Part model, mm, in its own coordinate system. Face numbers are marked on the shaded views. Round coordinates to 2 decimals unless told otherwise and drop trailing zeros. Order: outer loops, then holes, each group sorted by start corner. A loop starts at its lowest first (then second) coordinate and runs counter-clockwise, first axis right, second up. Notation, with made-up numbers: M 74.5,48.25 L 106.5,48.25 A15 ccw 106.5,66.25 Z; hole C 73,-15 d3. An arc over 180 degrees is marked long. Write each question's results on one line, items separated by ' | '. Start each with the question number.
1. Band-saw the part on C-C, the plane x = -30. List the corners of the cut face in (y, z) (3 decimals).
2. Probe L1, parallel to Y at x = 54.25, z = 6; L2, parallel to X at y = 16, z = 8; L3, parallel to Y at x = -25, z = 9. List the from-to ranges inside material, lowest first. Write a range as [from, to].
3. Two-plate mould, pull along Y, no slides. Class the marked faces 1, 2, 3 and 4: +Y half, -Y half, draft (parallel to the pull), parting line (faces both ways), or undercut.
4. Band-saw the part on A-A, the plane x = 55. List the corners of the cut face in (y, z), then the cut area to 3 significant figures.
5. Drop flat-ended pins along their axis: pin 1 Ø3 at (y, z) = (-20, 6.5) entering from +X; pin 2 Ø1 at (y, z) = (18, 10) entering from -X; pin 3 Ø0.9 at (x, z) = (-30, 6.5) entering from +Y. Give the stop position or say it passes through.
6. Band-saw the part on D-D, the plane z = 10.25. List the corners of the cut face in (x, y).
```python
from build123d import *

# Parameters (mm, degrees)
SKETCH1_W           = 130
SKETCH1_H           = 60
SKETCH1_R           = 8
SKETCH1_R_2         = 3.25
BOSS_EXTRUDE1_DEPTH = 12
FILLET1_R           = 6
SKETCH2_R           = 3
SKETCH2_R_2         = 2.5
CUT_EXTRUDE1_DEPTH  = 20
SKETCH3_R           = 3
SKETCH3_R_2         = 1.5
CUT_EXTRUDE2_DEPTH  = 15


with BuildPart() as part:
    # Sketch1 → Boss-Extrude1 (new body)
    with BuildSketch(Plane.XY):
        Rectangle(SKETCH1_W, SKETCH1_H)
        with Locations((-25, 0)):
            Circle(SKETCH1_R, mode=Mode.SUBTRACT)
        with Locations((-5.554563517, 19.445436483)):
            Circle(SKETCH1_R_2, mode=Mode.SUBTRACT)
        with Locations((-44.445436483, 19.445436483)):
            Circle(SKETCH1_R_2, mode=Mode.SUBTRACT)
        with Locations(Location((-44.445436483, -19.445436483, 0), (0, 0, 180))):
            Circle(SKETCH1_R_2, mode=Mode.SUBTRACT)
        with Locations(Location((-5.554563517, -19.445436483, 0), (0, 0, 180))):
            Circle(SKETCH1_R_2, mode=Mode.SUBTRACT)
    extrude(amount=BOSS_EXTRUDE1_DEPTH)

    # Fillet1
    fillet1_edges = [part.edges().sort_by_distance(p)[0] for p in [
        (-65, 0, 0),
        (-65, 0, 12),
    ]]
    fillet(fillet1_edges, radius=FILLET1_R - 0.0001)  # a hair under: the kernel refuses the full size

    # Sketch2 → Cut-Extrude1 (cut)
    with BuildSketch(Plane(origin=(65, 0, 0), x_dir=(0, 0, -1), z_dir=(1, 0, 0))):
        with Locations((-6, 20)):
            Circle(SKETCH2_R)
        with Locations((-6, 10)):
            Circle(SKETCH2_R_2)
        with Locations(Location((-6, -10, 0), (0, 0, 180))):
            Circle(SKETCH2_R_2)
        with Locations(Location((-6, -20, 0), (0, 0, 180))):
            Circle(SKETCH2_R)
    extrude(amount=-CUT_EXTRUDE1_DEPTH, mode=Mode.SUBTRACT)

    # Sketch3 → Cut-Extrude2 (cut)
    with BuildSketch(Plane(origin=(0, 30, 0), x_dir=(1, 0, 0), z_dir=(0, 1, 0))):
        with Locations(Location((-13, -6, 0), (0, 0, 270))):
            Circle(SKETCH3_R)
        with Locations(Location((-20, -6, 0), (0, 0, 270))):
            Circle(SKETCH3_R_2)
        with Locations(Location((-30, -6, 0), (0, 0, 90))):
            Circle(SKETCH3_R_2)
        with Locations(Location((-37, -6, 0), (0, 0, 90))):
            Circle(SKETCH3_R)
    extrude(amount=-CUT_EXTRUDE2_DEPTH, mode=Mode.SUBTRACT)


solid = part.part
```
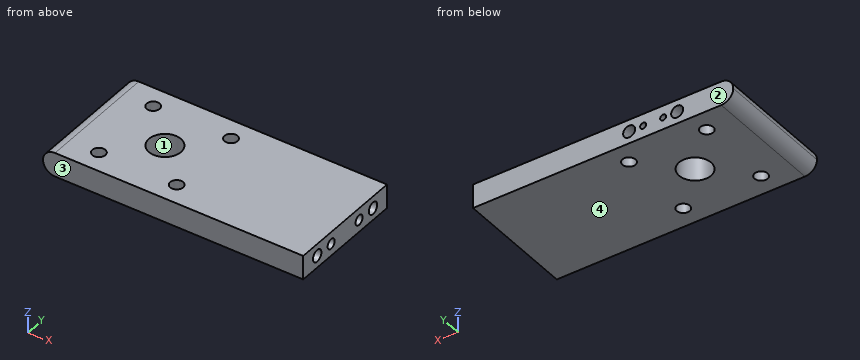
Solution:
1) outline: M -30,0 L -6.245,0 L -6.245,12 L -30,12 Z; M 6.245,0 L 30,0 L 30,4.5 L 15,4.5 L 15,7.5 L 30,7.5 L 30,12 L 6.245,12 Z
2) L1: [-30, -23], [-17, -12.5], [-7.5, 7.5], [12.5, 17], [23, 30] | L2: [-64.66, -39.24], [-34.76, -15.24], [-10.76, 65] | L3: [-30, -8], [8, 30]
3) face 1: undercut | face 2: +Y half | face 3: -Y half | face 4: draft
4) outline: M -30,0 L 30,0 L 30,12 L -30,12 Z; hole C -20,6 d6; hole C -10,6 d5; hole C 10,6 d5; hole C 20,6 d6 | area: 624 mm^2
5) pin 1: x = 45 | pin 2: x = -63.87 | pin 3: y = 15
6) outline: M -63.24,-30 L 65,-30 L 65,30 L -63.24,30 Z; hole C -44.45,-19.45 d6.5; hole C -44.45,19.45 d6.5; hole C -25,0 d16; hole C -5.55,-19.45 d6.5; hole C -5.55,19.45 d6.5
